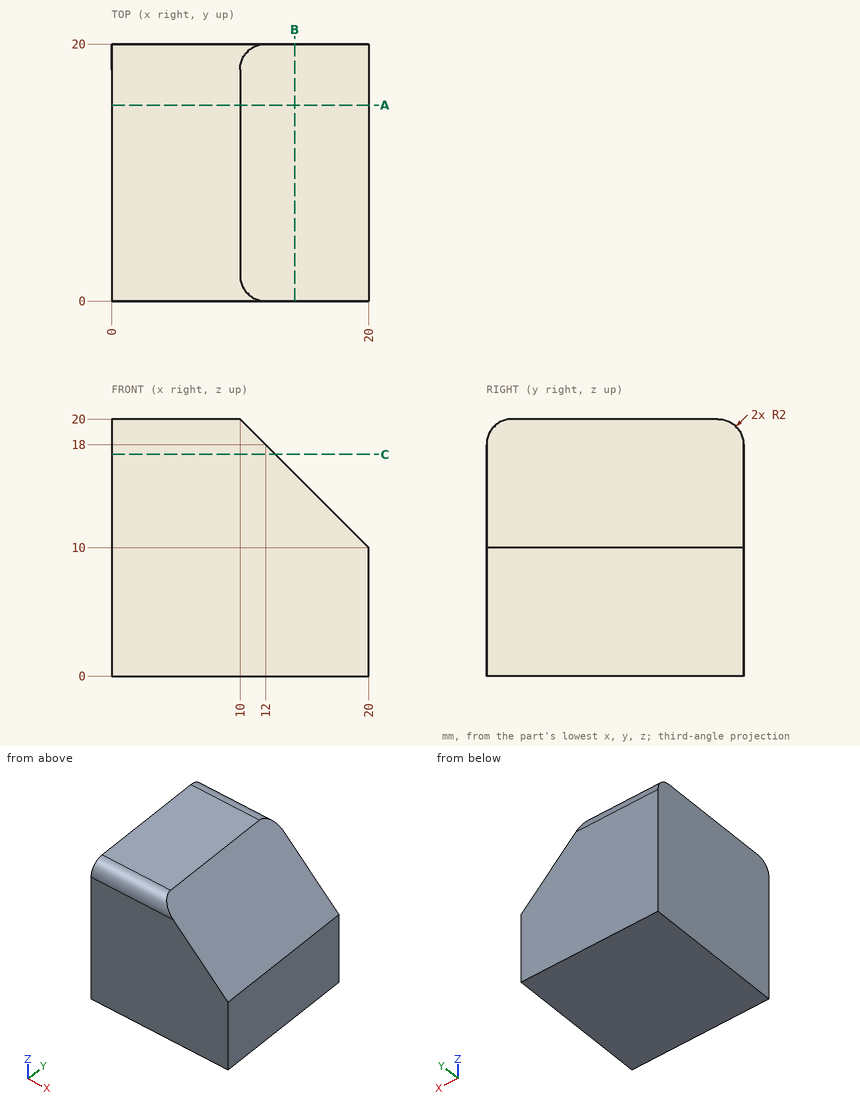
Could you check a few things on this drawing? It's one solid part, dimensions in mm from its lowest x, y, z. Round coordinates to 2 decimals unless told otherwise and drop trailing zeros. Write each loop counter-clockwise with the first axis right and the second up, starting at its lowest first coordinate (ties: lowest second). Pieces come first, ordered by that corner, then holes. Notation, with made-up numbers: (59.25, -16) -> (96.25, -16) arc R18 cw to (96.25, 6) -> close; hole circle Ø3 at (66.5, -39). An arc over 180 degrees is marked (long way). Use a Markdown table: item, result.
1. If we section it at B-B (x = 14.25): List the corners of the cut face in (y, z) for me, then the cut area to 3 significant figures.
Answer key:
| item | result |
|---|---|
| outline | (0, 0) -> (20, 0) -> (20, 15.75) -> (0, 15.75) -> close |
| area | 315 mm^2 |
2. If we section it at A-A (y = 15.25): List the corners of the cut face in (x, z) for me, then the cut area to 3 significant figures.
Answer key:
| item | result |
|---|---|
| outline | (0, 0) -> (20, 0) -> (20, 10) -> (10, 20) -> (0, 20) -> close |
| area | 350 mm^2 |
3. Please list where these lines run through material, in increasing order: probe 1 along X at (y, z) = (6.5, 12); probe 2 along X at (y, z) = (2.75, 12.5); probe 3 along Z at (x, y) = (11.5, 7.75).
Answer key:
| item | result |
|---|---|
| probe 1 | x = 0 to 18 |
| probe 2 | x = 0 to 17.5 |
| probe 3 | z = 0 to 18.5 |
4. If we section it at C-C (z = 17.25): List the corners of the cut face in (x, y) for me.
Answer key:
| item | result |
|---|---|
| outline | (0, 0) -> (12.75, 0) -> (12.75, 20) -> (0, 20) -> close |
5. For pin 1 Ø5 at (y, z) = (10, 14.5) entering from +X; pin 2 Ø1.5 at (y, z) = (15.5, 14) entering from +X, each with a flat end and sliding along its axis, tell me the tip position at first contact or that it passes through.
Answer key:
| item | result |
|---|---|
| pin 1 | stops at x = 18 |
| pin 2 | stops at x = 16.75 |
